Here's how the part is built. I have some questions about the finished solid (model axes, mm). Face numbers are marked on the shaded views. A direction names the side the tool comes from. Coordinates: 2 decimals unless noted, no trailing zeros. Loops run counter-clockwise (first coordinate to the right, second up) from the corner with the lowest first, then second, coordinate; pieces in that order, holes last. Notation, with made-up numbers: (68, 6.5) - (91, 6.5) arc R14 cw to (91, 11.5) - close; hole circle Ø2 at (20, 88). An arc over 180 degrees is marked (long way). Use a Markdown table: item, result.
```python
from build123d import *

# Parameters (mm, degrees)
F0_W     = 45
F0_H     = 350
F2_DEPTH = 45
F1_W     = 135
F1_H     = 45
F3_DEPTH = 45


with BuildPart() as f2:
    # F0 (on Top) → F2 (new body)
    with BuildSketch(Plane.XY):
        with Locations((112.5, 175)):
            Rectangle(F0_W, F0_H)
    extrude(amount=F2_DEPTH)



with BuildPart() as f2b:
    # F0 (on Top) → F2, piece 2 (new body)
    with BuildSketch(Plane.XY):
        with Locations((37.5, 175)):
            Rectangle(F0_W, F0_H)
    extrude(amount=F2_DEPTH)


with BuildPart() as f3:
    # F1 (on Top) → F3 (new body)
    with BuildSketch(Plane.XY):
        with Locations((67.5, 237.5)):
            Rectangle(F1_W, F1_H)
    extrude(amount=-F3_DEPTH)


with BuildPart() as f2_1:
    add(f2.part)

    add(f2b.part)  # F4 merges F2b
    # F4: F3, F2b, F2 across plane
    add(f3.part.mirror(Plane.XZ))
    add(f2b.part.mirror(Plane.XZ))
    add(f2.part.mirror(Plane.XZ))



with BuildPart() as f2_2:
    add(f2_1.part)

    add(f3.part)  # F5 merges F3
    # F5: F2, F3 across plane
    add(f2_1.part.mirror(Plane.YZ))
    add(f3.part.mirror(Plane.YZ))


solid = f2_2.part
```
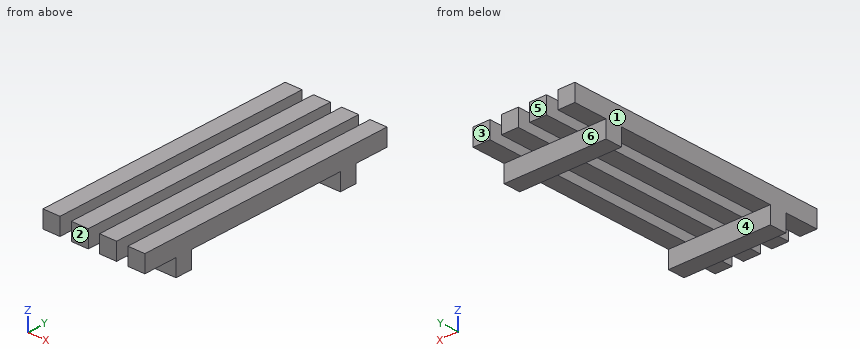
Q1. If we mould it in two halves opening along Y, with no side actions, what happens to the marked faces 1, 2, 3 and 4? For each: pulls with the +Y half, pulls with the -Y half, needs draft (parallel to the pull), parting line crosses it, or undercut.
Check values:
| item | result |
|---|---|
| face 1 | needs draft |
| face 2 | pulls with the -Y half |
| face 3 | pulls with the +Y half |
| face 4 | undercut |
Q2. I want a section at C-C, the plane z = 35. Write out the boundary of the cut face in (x, y).
Check values:
| item | result |
|---|---|
| outline | (-135, -350) - (-90, -350) - (-90, 350) - (-135, 350) - close; (-60, -350) - (-15, -350) - (-15, 350) - (-60, 350) - close; (15, -350) - (60, -350) - (60, 350) - (15, 350) - close; (90, -350) - (135, -350) - (135, 350) - (90, 350) - close |
Q3. Please list where these lines run through material, in increasing order: L1, parallel to X at y = 220, z = 28; L2, parallel to Y at x = 96.5, z = -24; L3, parallel to Z at x = 115.5, y = 136. Write a range as from..to.
Check values:
| item | result |
|---|---|
| L1 | -135..-90, -60..-15, 15..60, 90..135 |
| L2 | -260..-215, 215..260 |
| L3 | 0..45 |
Q4. I want a section at D-D, the plane x = -105.5. Write out the boundary of the cut face in (y, z).
Check values:
| item | result |
|---|---|
| outline | (-350, 0) - (-260, 0) - (-260, -45) - (-215, -45) - (-215, 0) - (215, 0) - (215, -45) - (260, -45) - (260, 0) - (350, 0) - (350, 45) - (-350, 45) - close |
Q5. Will these pins go through, and if not, where does the flat tip stop? P1, Ø13.5, axis at x = 102.5, y = -90.5, coming from the -Z side; P2, Ø4, axis at x = -95.5, z = -30, coming from the +Y side; P3, Ø9, axis at x = -80, y = 243.5, coming from the +Z side.
Check values:
| item | result |
|---|---|
| P1 | z = 0 |
| P2 | y = 260 |
| P3 | z = 0 |
Q6. I want a section at B-B, the plane y = 171. Write out the boundary of the cut face in (x, z).
Check values:
| item | result |
|---|---|
| outline | (-135, 0) - (-90, 0) - (-90, 45) - (-135, 45) - close; (-60, 0) - (-15, 0) - (-15, 45) - (-60, 45) - close; (15, 0) - (60, 0) - (60, 45) - (15, 45) - close; (90, 0) - (135, 0) - (135, 45) - (90, 45) - close |
Q7. Which directions (+Z, -Z, +X, -X, +Y, -Y) give clear straight access to the entire face, cutting with the end or side of a thin tool? Please do the marked faces 5 and 6.
Check values:
| item | result |
|---|---|
| face 5 | +Z, -Z, +X, -X, +Y |
| face 6 | -Z, +X, -X, +Y |
Q8. I want a section at A-A, the plane z = -28. Write out the boundary of the cut face in (x, y), then the cut area to 3 significant figures.
Check values:
| item | result |
|---|---|
| outline | (-135, -260) - (135, -260) - (135, -215) - (-135, -215) - close; (-135, 215) - (135, 215) - (135, 260) - (-135, 260) - close |
| area | 24,300 mm^2 |
